For this review, take the finished solid that the model builds, in its own axes (mm). Coordinates: 2 decimals unless noted, no trailing zeros. Loops run counter-clockwise (first coordinate to the right, second up) from the corner with the lowest first, then second, coordinate; pieces in that order, holes last.
1. Mouldability with a two-part tool opening along X and no side actions: class faces 1 (the face through (38.506, 1.479, -0.264)), 2 (the face through (-38.506, 1.479, -0.264)), 3 (the face through (-1, 0, 68)), 4 (the face through (-62.15, 1.52, -56.99)) as pulls with the +X half, pulls with the -X half, needs draft (parallel to the pull), parting line crosses it, or undercut.
2. Clearance check with a flat-ended pin moving along its axis: P1, Ø1.5, axis at x = -42.5, z = 91, coming from the -Y side. State where the tip first meets the part, or that it passes through.
3. To check wall thickness, follow probe 1 along Z at (x, y) = (-44.5, 1.75); probe 2 along Z at (x, y) = (49, 0.75); probe 3 along Z at (x, y) = (-57, 0.7). State the ranges of each line that lie inside material, in increasing order.
4. Take a section at B-B, the plane x = -44.5. State the section outline as (y, z) points, then the cut area to 3 significant figures.
5. Take a section at A-A, the plane z = 0. State the section outline as (x, y) points, then the cut area to 3 significant figures.
```python
from build123d import *

# Parameters (mm, degrees)
SKETCH1_W           = 130
SKETCH1_H           = 120
BOSS_EXTRUDE1_DEPTH = 3
CUT_EXTRUDE1_START  = -4
SKETCH2_R           = 6
CUT_EXTRUDE1_DEPTH  = 5
SKETCH3_W           = 130
SKETCH3_H           = 3
BOSS_EXTRUDE2_DEPTH = 140
FILLET1_R           = 10


with BuildPart() as part:
    # Sketch1 → Boss-Extrude1 (new body)
    with BuildSketch(Plane(origin=(0, 0, 0), x_dir=(1, 0, 0), z_dir=(0, 1, 0))):
        Rectangle(SKETCH1_W, SKETCH1_H)
    extrude(amount=BOSS_EXTRUDE1_DEPTH)

    # Sketch2 → Cut-Extrude1 (cut)
    with BuildSketch(Plane(origin=(0, 3, 0), x_dir=(1, 0, 0), z_dir=(0, 1, 0)).offset(CUT_EXTRUDE1_START)):
        with Locations((44.5, 0)):
            Circle(SKETCH2_R)
    cut_extrude1 = extrude(amount=CUT_EXTRUDE1_DEPTH, mode=Mode.SUBTRACT)

    # Mirror1: Cut-Extrude1 across plane
    add(cut_extrude1.mirror(Plane(origin=(0, 0, 0), x_dir=(0, 0, 1), z_dir=(1, 0, 0))), mode=Mode.SUBTRACT)

    # Sketch3 → Boss-Extrude2 (add)
    with BuildSketch(Plane.XY.offset(60)):
        with Locations((0, 1.5)):
            Rectangle(SKETCH3_W, SKETCH3_H)
    extrude(amount=BOSS_EXTRUDE2_DEPTH)

    # Fillet1
    fillet1_edges = [part.edges().sort_by_distance(p)[0] for p in [
        (-65, 1.5, 200),
        (65, 1.5, 200),
        (-65, 1.5, -60),
        (65, 1.5, -60),
    ]]
    fillet(fillet1_edges, radius=FILLET1_R)


solid = part.part
```
Results list:
1. face 1: undercut
1. face 2: undercut
1. face 3: needs draft
1. face 4: pulls with the -X half
2. P1: stops at y = 0
3. probe 1: z = -60 to -6, 6 to 200
3. probe 2: z = -60 to -3.97, 3.97 to 200
3. probe 3: z = -59.8 to 199.8
4. outline: (0, -60) - (3, -60) - (3, -6) - (0, -6) - close; (0, 6) - (3, 6) - (3, 200) - (0, 200) - close
4. area: 744 mm2
5. outline: (-65, 0) - (-50.5, 0) - (-50.5, 3) - (-65, 3) - close; (-38.5, 0) - (38.5, 0) - (38.5, 3) - (-38.5, 3) - close; (50.5, 0) - (65, 0) - (65, 3) - (50.5, 3) - close
5. area: 318 mm2
